Geometry: final body of the model. Coordinates: model frame, mm. A direction names the side the tool comes from. Give positions to 0.01 mm unless a question says otherwise; leave off trailing zeros. Order: outer loops, then holes, each group sorted by start corner. A loop starts at its lowest first (then second) coordinate and runs counter-clockwise, first axis right, second up. Notation, with made-up numbers: (50, 7.25) - (66, 7.25) arc R18 cw to (66, 35.25) - close; hole circle Ø10 at (20, -16.5). An arc over 180 degrees is marked (long way). Use one line per item in the form item = value.
from build123d import *

# Parameters (mm, degrees)
CHAMFER_1_SIZE      = 2.195
SKETCH_2_R          = 37.5
CUT_EXTRUDE_1_DEPTH = 18
SKETCH_3_R          = 25
EXTRUDE_1_DEPTH     = 17


with BuildPart() as part:
    # Эскиз1 → Повернуть1 (revolve)
    with BuildSketch(Plane.XY):
        Polygon((25, 0), (32, 0), (32, 20), (28, 20), (28, 24), (37.5, 24), (37.5, 29), (32.5, 29), (32.5, 42.535898385), (26.5, 46), (19, 46), (19, 5), (25, 5), align=None)
    revolve(axis=Axis((0, 57.260780425, 0), (0, -1, 0)))

    # Фаска1
    chamfer_1_edges = [part.edges().sort_by_distance(p)[0] for p in [
        (-32, 0, 0),
    ]]
    chamfer(chamfer_1_edges, length=CHAMFER_1_SIZE)

    # Эскиз2 → Вырез-Вытянуть1 (cut, through all)
    with BuildSketch(Plane(origin=(0, 29, 0), x_dir=(1, 0, 0), z_dir=(0, 1, 0))):
        Circle(SKETCH_2_R)
        Polygon((0, 34.641016151), (-30, 17.320508076), (-30, -17.320508076), (0, -34.641016151), (30, -17.320508076), (30, 17.320508076), align=None, mode=Mode.SUBTRACT)
    extrude(amount=CUT_EXTRUDE_1_DEPTH, mode=Mode.SUBTRACT)

    # Эскиз3 → Бобышка-Вытянуть1 (add)
    with BuildSketch(Plane(origin=(0, 29, 0), x_dir=(1, 0, 0), z_dir=(0, 1, 0))):
        Polygon((0, 34.641016151), (-30, 17.320508076), (-30, -17.320508076), (0, -34.641016151), (30, -17.320508076), (30, 17.320508076), align=None)
        Circle(SKETCH_3_R, mode=Mode.SUBTRACT)
    extrude(amount=EXTRUDE_1_DEPTH)

    # Эскиз4 → Вырез-Повернуть1 (revolve, cut)
    with BuildSketch(Plane.XY):
        Polygon((-30, 46), (-45, 46), (-45, 37.339745962), align=None)
    revolve(axis=Axis((0, 0, 0), (0, 1, 0)), mode=Mode.SUBTRACT)


solid = part.part
(1) Ray query, line 1 along Z through (x, y) = (0, 3.6); line 2 along Z through (x, y) = (0, 14); line 3 along Y through (x, z) = (29, -19). Return the intervals inside material, ascending.
Computed values:
line_1 = -32 to -25, 25 to 32
line_2 = -32 to -19, 19 to 32
line_3 = 24 to 29
(2) Pull-direction query (Y, two-part tool) for faces 5 (the face through (28, 24, -3)), 6 (the face through (15.21, 37.38, -25.86)), 7 (the face through (26.9, 45.36, 15.62)); classes: released by +Y, released by -Y, zero draft, split by the parting line, or undercut.
Computed values:
face_5 = undercut
face_6 = zero draft
face_7 = released by +Y
(3) Reachability of faces 1 (the face through (14.79, 37.38, 26.1)), 2 (the face through (-14.79, 37.38, -26.1)), 3 (the face through (30, 37, 0)), 4 (the face through (4, 5, 19)) from +Z, -Z, +X, -X, +Y, -Y: full face, straight path, thin tool, end or side. Return the list, or none.
Computed values:
face_1 = +Z, +X, +Y
face_2 = -Z, -X, +Y
face_3 = +Z, -Z, +X, +Y
face_4 = -Y
(4) Cut plane A-A on y = 41. Output: boundary loops of the cut face in (x, z), plus the area to 3 significant figures.
Computed values:
outline = (-30, -17.32) - (0, -34.64) - (30, -17.32) - (30, 17.32) - (0, 34.64) - (-30, 17.32) - close; hole circle Ø38 at (0, 0)
area = 1,980 mm²
(5) Contact query for flat-ended pins moving along their axis: pin 1 Ø8.5 at (y, z) = (35, 6) entering from -X; pin 2 Ø22.5 at (x, z) = (11, 7) entering from -Y; pin 3 Ø15 at (x, z) = (9.5, -0.5) entering from -Y; pin 4 Ø8 at (x, z) = (-30, -21) entering from +Y. Output: stop coordinate, or through.
Computed values:
pin_1 = -30
pin_2 = 5
pin_3 = through
pin_4 = 44.49
